```python
from build123d import *

# Parameters (mm, degrees)
SKETCH006_R   = 43
SKETCH006_R_2 = 1.5
SKETCH006_R_3 = 9
PAD_DEPTH     = 1.5
CHAMFER_SIZE  = 1.4


with BuildPart() as part:
    # Sketch006 → Pad (new body)
    with BuildSketch(Plane.XY.offset(22)):
        Circle(SKETCH006_R)
        with Locations((0, 36)):
            Circle(SKETCH006_R_2, mode=Mode.SUBTRACT)
        with Locations((31.176915, -18)):
            Circle(SKETCH006_R_2, mode=Mode.SUBTRACT)
        with Locations((-31.176915, -18)):
            Circle(SKETCH006_R_2, mode=Mode.SUBTRACT)
        Circle(SKETCH006_R_3, mode=Mode.SUBTRACT)
    extrude(amount=PAD_DEPTH)

    # Chamfer
    chamfer_edges = [part.edges().sort_by_distance(p)[0] for p in [
        (-32.676915, -18, 22),
        (-1.5, 36, 22),
        (29.676915, -18, 22),
    ]]
    chamfer(chamfer_edges, length=CHAMFER_SIZE)


solid = part.part
```
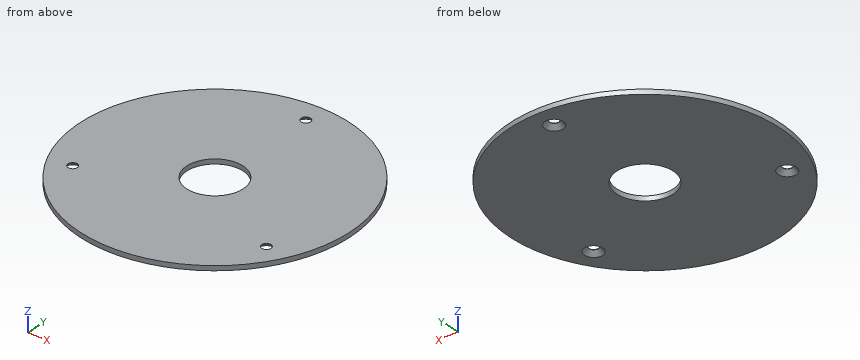
Build history of the part. All positions in model axes, mm. Give positions to 0.01 mm unless a question says otherwise; leave off trailing zeros. Loops run counter-clockwise (first coordinate to the right, second up) from the corner with the lowest first, then second, coordinate; pieces in that order, holes last. Notation, with made-up numbers: (54.5, 41.5) -> (69.5, 41.5) arc R31 cw to (69.5, 70.5) -> close; hole circle Ø10 at (24.5, -11.5). An arc over 180 degrees is marked (long way). One line per question, with ' | ' between items. Start each with the question number.
1) Pin check, flat tips, straight feed: pin 1 (4 mm diameter, centred on x = 31.18, y = -18, fed in from +Z); pin 2 (4 mm diameter, centred on x = 0, y = 36, fed in from -Z). Stop position of each tip, or through.
2) Probe L1, parallel to Y at x = 0, z = 23.4; L2, parallel to Y at x = 1, z = 22.3; L3, parallel to Y at x = 3, z = 22.75. List the from-to ranges inside material, lowest first.
3) Cut at B-B (x = 0). Give the cut face in (y, z), plus the area to 3 significant figures.
4) Cut at D-D (z = 22.35). Give the cut face in (x, y), plus the area to 3 significant figures.
5) Cut at C-C (y = -18). Give the cut face in (x, z).
6) Cut at A-A (y = 0). Give the cut face in (x, z), plus the area to 3 significant figures.
Return value:
1) pin 1: z = 23.5 | pin 2: z = 22.9
2) L1: -43 to -9, 9 to 34.5, 37.5 to 43 | L2: -42.99 to -8.94, 8.94 to 33.6, 38.4 to 42.99 | L3: -42.9 to -8.49, 8.49 to 42.9
3) outline: (-43, 22) -> (-9, 22) -> (-9, 23.5) -> (-43, 23.5) -> close; (9, 22) -> (33.1, 22) -> (34.5, 23.4) -> (34.5, 23.5) -> (9, 23.5) -> close; (37.5, 23.4) -> (38.9, 22) -> (43, 22) -> (43, 23.5) -> (37.5, 23.5) -> close | area: 95.5 mm^2
4) outline: circle Ø86 at (0, 0); hole circle Ø5.1 at (-31.18, -18); hole circle Ø18 at (0, 0); hole circle Ø5.1 at (0, 36); hole circle Ø5.1 at (31.18, -18) | area: 5,490 mm^2
5) outline: (-39.05, 22) -> (-34.08, 22) -> (-32.68, 23.4) -> (-32.68, 23.5) -> (-39.05, 23.5) -> close; (-29.68, 23.4) -> (-28.28, 22) -> (28.28, 22) -> (29.68, 23.4) -> (29.68, 23.5) -> (-29.68, 23.5) -> close; (32.68, 23.4) -> (34.08, 22) -> (39.05, 22) -> (39.05, 23.5) -> (32.68, 23.5) -> close
6) outline: (-43, 22) -> (-9, 22) -> (-9, 23.5) -> (-43, 23.5) -> close; (9, 22) -> (43, 22) -> (43, 23.5) -> (9, 23.5) -> close | area: 102 mm^2
